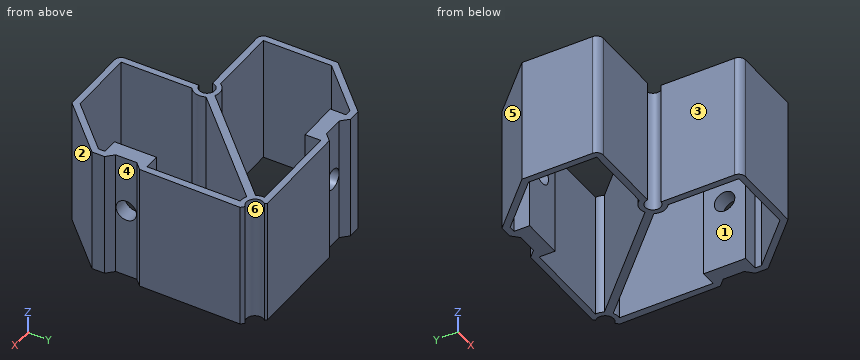
Autodesk Inventor part; units mm, degrees
ref_plane "Work Plane1" through (4.2657, -41.0804, 0) normal (1, 0, 0) x (0, 0, -1)
ref_plane "Work Plane2" through (-28.6911, -33.1074, 0) normal (0.7071, -0.7071, 0) x (-0.7071, -0.7071, 0)
ref_plane "Plano de trabajo3" through (0, 0, -18.5) normal (0, 0, 1) x (1, 0, 0)
sketch "Sketch1" plane through (0, 0, 0) normal (0, 0, 1) x (1, 0, 0)
  line L0 (0, 0) -> (-27.4191, 0)
  line L1 (-27.4191, 0) -> (-27.4191, -4.6)
  line L2 (-27.4191, -4.6) -> (-39.7191, -4.6)
  line L3 (-39.7191, -4.6) -> (-39.7191, 0)
  line L4 (-39.7191, 0) -> (-41.6191, 0)
  line L5 (-55.1956, -13.5765) -> (-41.6191, 0)
  line L6 (-55.1956, -33.5765) -> (-55.1956, -13.5765)
  line L7 (-34.3956, -33.5765) -> (-55.1956, -33.5765)
  line L8 (1.6418, 1.9) -> (-28.4235, 1.9)
  line L9 (-28.4235, 1.9) -> (-30.4741, -0.1506)
  line L10 (-30.4741, -0.1506) -> (-36.6641, -0.1506)
  line L11 (-36.6641, -0.1506) -> (-38.7147, 1.9)
  line L12 (-42.4061, 1.9) -> (-38.7147, 1.9)
  line L13 (-57.3968, -13.0907) -> (-42.4061, 1.9)
  line L14 (-57.0956, -33.4765) -> (-57.0956, -12.7894)
  line L15 (-33.5097, -35.4765) -> (-55.0956, -35.4765)
  arc A0 (-57.0956, -33.4765) -> (-55.0956, -35.4765) centre (-55.0956, -33.4765) ccw
  line L16 (-29.5043, -32.2942) -> (0.4547, -2.3353)
  line L17 (8.0118, 3.5954) -> (-35.5125, -39.9288) construction
  line L18 (4.4163, -4.4163) -> (4.4163, -31.8354)
  line L19 (4.4163, -31.8354) -> (-0.1837, -31.8354)
  line L20 (-0.1837, -31.8354) -> (-0.1837, -44.1354)
  line L21 (-0.1837, -44.1354) -> (4.4163, -44.1354)
  line L22 (4.4163, -44.1354) -> (4.4163, -46.0354)
  line L23 (-9.1601, -59.6119) -> (4.4163, -46.0354)
  line L24 (-29.1601, -59.6119) -> (-9.1601, -59.6119)
  line L25 (-29.1601, -38.8119) -> (-29.1601, -59.6119)
  line L26 (6.6743, -3.1325) -> (6.3163, -32.8398)
  line L27 (6.3163, -32.8398) -> (4.2657, -34.8904)
  line L28 (4.2657, -34.8904) -> (4.2657, -41.0804)
  line L29 (4.2657, -41.0804) -> (6.3163, -43.131)
  line L30 (6.3163, -46.8224) -> (6.3163, -43.131)
  line L31 (-8.6743, -61.8131) -> (6.3163, -46.8224)
  line L32 (-29.0601, -61.5119) -> (-8.3731, -61.5119)
  line L33 (-31.0601, -37.926) -> (-31.0601, -59.5119)
  arc A1 (-31.0601, -59.5119) -> (-29.0601, -61.5119) centre (-29.0601, -59.5119) ccw
  line L34 (-27.8779, -33.9206) -> (2.081, -3.9617)
  arc A2 (-29.1601, -38.8119) -> (-27.8779, -33.9206) centre (-31.2373, -35.6537) ccw
  arc A3 (-29.5043, -32.2942) -> (-34.3956, -33.5765) centre (-31.2373, -35.6537) ccw
  arc A4 (2.081, -3.9617) -> (4.4163, -4.4163) centre (3.9791, -0.4372) ccw
  arc A5 (0, 0) -> (0.4547, -2.3353) centre (3.9791, -0.4372) ccw
  arc A6 (2.2092, 1.3327) -> (5.749, -2.2072) centre (3.9791, -0.4372) ccw
  arc A7 (-31.0601, -37.926) -> (-33.5097, -35.4765) centre (-31.2373, -35.6537) ccw
  line L35 (1.6418, 1.9) -> (2.2092, 1.3327)
  line L36 (5.749, -2.2072) -> (6.6743, -3.1325)
  point P0 (0, 0)
  point P1 (-57.0956, -35.4765)
  point P2 (-13.7504, -18.1667)
  point P3 (-31.0601, -61.5119)
  point P4 (-29.6257, -34.042)
  dimension "d1" = 4.6
  dimension "d2" = 12.3
  dimension "d3" = 1.9
  dimension "d4" = 135
  dimension "d5" = 19.2
  dimension "d6" = 20
  dimension "d7" = 20.8
  dimension "d10" = 1.9
  dimension "d11" = 2.9
  dimension "d12" = 2.9
  dimension "d14" = 6.19
  dimension "d15" = 3.055
  dimension "d17" = 135
  dimension "d18" = 135
  dimension "d20" = 21.2
  dimension "d22" = 1.9
  dimension "d23" = 1.9
  dimension "d24" = 1.9
  dimension "d25" = 22.687
  dimension "d27" = 2
  dimension "d33" = 2.3
  dimension "d34" = 90
  dimension "d45" = 1.5
  dimension "d46" = 1.5009
extrude "Extrusion1" add sketch "Sketch1" against normal blind 37
ref_plane "Work Plane1" through (4.2657, -41.0804, 0) normal (1, 0, 0) x (0, 0, -1)
sketch "Sketch2" plane through (4.2657, -41.0804, 0) normal (1, 0, 0) x (0, 0, -1)
  circle A0 centre (16.5, 3.095) radius 3
  line L0 (0, 0) -> (0, 6.19)
  line L1 (0, 0) -> (37, 0)
  point P0 (0, 41.0804)
  dimension "d52" = 6
  dimension "d53" = 16.5
  dimension "d55" = 3.095
extrude "Extrusion2" cut sketch "Sketch2" against normal blind 10
thread "Thread1"
ref_plane "Work Plane2" through (-28.6911, -33.1074, 0) normal (0.7071, -0.7071, 0) x (-0.7071, -0.7071, 0)
mirror "Mirror1" about plane through (-28.6911, -33.1074, 0) normal (0.7071, -0.7071, 0) of "Extrusion2"
ref_plane "Plano de trabajo3" through (0, 0, -18.5) normal (0, 0, 1) x (1, 0, 0)
properties part number "ESCUADRA UNIÓN 45 GORDA"
Geometry check sheet. Reference: the model listing, model coordinates, mm. Face numbers are marked on the shaded views. A direction names the side the tool comes from. Coordinates: 2 decimals unless noted, no trailing zeros. Order: outer loops, then holes, each group sorted by start corner. A loop starts at its lowest first (then second) coordinate and runs counter-clockwise, first axis right, second up. Notation, with made-up numbers: (-3, -33.5) - (11, -33.5) arc R17 ccw to (11, -25.5) - close; hole circle Ø5 at (64.25, 74.5). An arc over 180 degrees is marked (long way). Answer in a Markdown table with one row per item. Add a question column.
1. Draft check along X on the marked faces 4, 5 and 6. Enter one of: +X half, -X half, draft (parallel to the pull), parting line (faces both ways), or undercut.
2. Section check A-A (y = -45). Enter the section's corners in (x, z), plus the area to 3 significant figures.
3. Section check B-B (x = -10.5). Enter the section's corners in (y, z), plus the area to 3 significant figures.
4. Gauge pin test, flat ends, axial feed: pin 1 Ø1.9 at (x, z) = (-32, -9.5) entering from +Y; pin 2 Ø1.4 at (x, z) = (2.5, -20.5) entering from -Y; pin 3 Ø1.9 at (y, z) = (-37, -21) entering from +X. Record the tip position at first contact, or that the pin passes through.
5. Section check D-D (z = -7). Give the number of separate pieces and of enclosed holes in the cut face, plus the area to 3 significant figures.
6. Access from +Z, -Z, +X, -X, +Y, -Y to the whole of each face (thin tool, end or side, straight path). Record for the marked faces 1, 2 and 3.
7. Section check C-C (y = -20.5). Enter the section's corners in (x, z) (3 decimals).
8. Material ranges on L1, parallel to Y at x = -7.5, z = -34; L2, parallel to X at y = -4.5, z = -21.5; L3, parallel to X at y = -10.5, z = -21.5, recorded low to high. Write a range as [from, to].
Data:
| question | item | result |
|---|---|---|
| 1 | face 4 | +X half |
| 1 | face 5 | -X half |
| 1 | face 6 | undercut |
| 2 | outline | (-31.06, -37) - (-29.16, -37) - (-29.16, 0) - (-31.06, 0) - close; (4.42, -37) - (6.32, -37) - (6.32, 0) - (4.42, 0) - close |
| 2 | area | 141 mm² |
| 3 | outline | (-61.51, -37) - (-59.61, -37) - (-59.61, 0) - (-61.51, 0) - close; (-16.54, -37) - (-13.29, -37) - (-13.29, 0) - (-16.54, 0) - close; (0, -37) - (1.9, -37) - (1.9, 0) - (0, 0) - close |
| 3 | area | 261 mm² |
| 4 | pin 1 | stops at y = -0.15 |
| 4 | pin 2 | stops at y = -51.34 |
| 4 | pin 3 | stops at x = 4.27 |
| 5 | separate pieces | 1 |
| 5 | enclosed holes | 2 |
| 5 | area | 615 mm² |
| 6 | face 1 | +Z, -Z |
| 6 | face 2 | +Z, -Z, +X, -Y |
| 6 | face 3 | +Z, -Z, -X, -Y |
| 7 | outline | (-57.096, -37) - (-55.196, -37) - (-55.196, 0) - (-57.096, 0) - close; (-17.71, -37) - (-14.457, -37) - (-14.457, 0) - (-17.71, 0) - close; (4.416, -37) - (6.465, -37) - (6.465, 0) - (4.416, 0) - close |
| 8 | L1 | y = [-60.64, -57.95], [-13.54, -10.29], [0, 1.9] |
| 8 | L2 | x = [-48.81, -46.12], [-39.72, -27.42], [-1.71, 1.54], [4.42, 6.66] |
| 8 | L3 | x = [-54.81, -52.12], [-7.71, -4.46], [4.42, 6.59] |
